The model under review builds one solid part; all positions refer to its coordinate system, in mm. Coordinates: 2 decimals unless noted, no trailing zeros. Order: outer loops, then holes, each group sorted by start corner. A loop starts at its lowest first (then second) coordinate and runs counter-clockwise, first axis right, second up. Notation, with made-up numbers: (-24.75, 2.5) -> (-12.75, 2.5) arc R18 ccw to (-12.75, 12.5) -> close; hole circle Ø3 at (26.25, 8.5). An arc over 180 degrees is marked (long way). Use one line per item in the form item = value. Start each with the question number.
(1) Insertion check: pin 1 Ø1 at (y, z) = (99.5, 3) entering from +X; pin 2 Ø1 at (y, z) = (52, 3.5) entering from +X. Each pin has a flat end and moves straight along its axis. Give the tip position at first contact, or say it passes through.
(2) Wall thickness on line 1 along X through (y, z) = (86.5, 4.75); line 2 along X through (y, z) = (78, 3.5); line 3 along Y through (x, z) = (342, 2): over which ranges is each line inside the solid? List them lowest first.
(3) Take a section at A-A (y = 76.2). State the section outline as (x, z) points.
(4) Take a section at C-C (y = 104.5). State the section outline as (x, z) points, then the cut area to 3 significant figures.
(5) Take a section at B-B (z = 2.25). State how many separate pieces and enclosed holes the cut face has, then the cut area to 3 significant figures.
```python
from build123d import *

# Parameters (mm, degrees)
LAYOUT_R            = 11.1125
LAYOUT_R_2          = 14.2875
BOSS_EXTRUDE1_DEPTH = 6.35


with BuildPart() as part:
    # Layout → Boss-Extrude1 (new body)
    with BuildSketch(Plane.XY):
        with BuildLine():
            Line((36.96482124, 44.45), (341.76482124, 44.45))
            ThreePointArc((341.76482124, 44.45), (359.725333482, 51.889487758), (367.16482124, 69.85))
            Line((367.16482124, 69.85), (367.16482124, 82.55))
            ThreePointArc((367.16482124, 82.55), (359.725333482, 100.510512242), (341.76482124, 107.95))
            Line((341.76482124, 107.95), (324.969720877, 107.95))
            Line((324.969720877, 107.95), (211.92127073, 107.95))
            Line((211.92127073, 107.95), (36.96482124, 107.95))
            ThreePointArc((36.96482124, 107.95), (19.004308998, 100.510512242), (11.56482124, 82.55))
            Line((11.56482124, 82.55), (11.56482124, 69.85))
            ThreePointArc((11.56482124, 69.85), (19.004308998, 51.889487758), (36.96482124, 44.45))
        make_face()
        with Locations((36.96482124, 76.2)):
            Circle(LAYOUT_R, mode=Mode.SUBTRACT)
        with Locations((341.76482124, 76.2)):
            Circle(LAYOUT_R_2, mode=Mode.SUBTRACT)
    extrude(amount=BOSS_EXTRUDE1_DEPTH)


solid = part.part
```
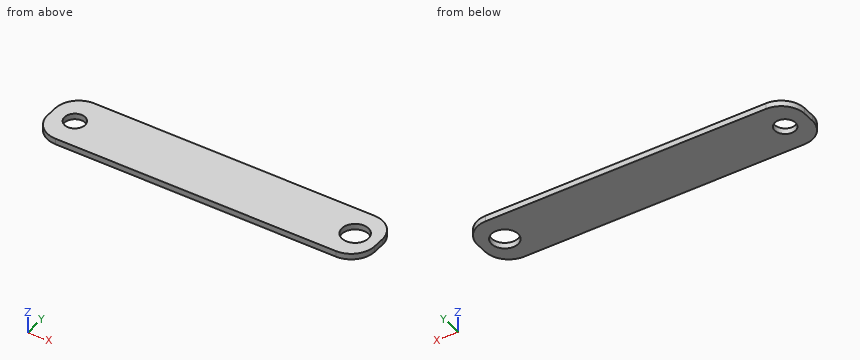
Findings:
q1.pin_1 = 361.12
q1.pin_2 = 360.32
q2.line_1 = 11.87 to 32.79, 41.14 to 331.86, 351.67 to 366.86
q2.line_2 = 11.56 to 26, 47.93 to 327.59, 355.94 to 367.16
q2.line_3 = 44.45 to 61.91, 90.49 to 107.95
q3.outline = (11.56, 0) -> (25.85, 0) -> (25.85, 6.35) -> (11.56, 6.35) -> close; (48.08, 0) -> (327.48, 0) -> (327.48, 6.35) -> (48.08, 6.35) -> close; (356.05, 0) -> (367.16, 0) -> (367.16, 6.35) -> (356.05, 6.35) -> close
q4.outline = (24.18, 0) -> (354.55, 0) -> (354.55, 6.35) -> (24.18, 6.35) -> close
q4.area = 2,100 mm²
q5.separate_pieces = 1
q5.enclosed_holes = 2
q5.area = 21,000 mm²
